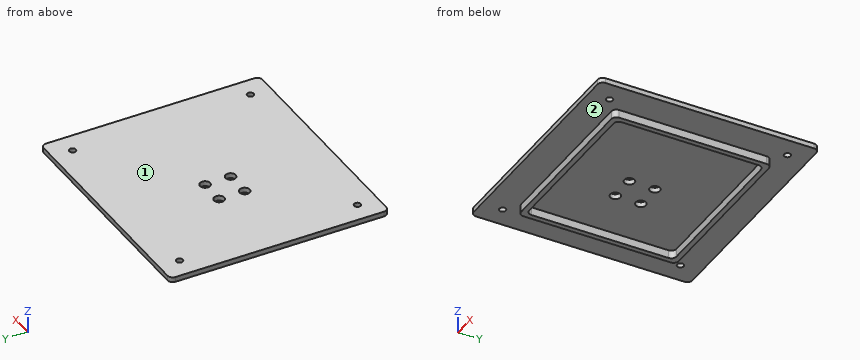
```python
from build123d import *

# Parameters (mm, degrees)
SKETCH_1_W                  = 170
SKETCH_1_H                  = 154.25
SKETCH_1_W_2                = 160
SKETCH_1_H_2                = 144.25
EXTRUDE_1_DEPTH             = 8
FILLET_1_R                  = 5
SKETCH_2_W                  = 230
SKETCH_2_H                  = 214.25
EXTRUDE_2_DEPTH             = 5
FILLET_2_R                  = 5
HOLE_WIZARD_6_4_6_4_1_D     = 6.4
HOLE_WIZARD_6_4_6_4_1_DEPTH = 5
HOLE_WIZARD_10_0_10_1_D     = 10


with BuildPart() as part:
    # 草图1 → 凸台-拉伸1 (new body)
    with BuildSketch(Plane.XY):
        Rectangle(SKETCH_1_W, SKETCH_1_H)
        Rectangle(SKETCH_1_W_2, SKETCH_1_H_2, mode=Mode.SUBTRACT)
    extrude(amount=EXTRUDE_1_DEPTH)

    # 圆角1
    fillet_1_edges = [part.edges().sort_by_distance(p)[0] for p in [
        (-80, 72.125, 4),
        (-80, -72.125, 4),
        (80, -72.125, 4),
        (80, 72.125, 4),
        (-85, 77.125, 4),
        (85, 77.125, 4),
        (85, -77.125, 4),
        (-85, -77.125, 4),
    ]]
    fillet(fillet_1_edges, radius=FILLET_1_R)

    # 草图2 → 凸台-拉伸2 (add)
    with BuildSketch(Plane.XY.offset(8)):
        Rectangle(SKETCH_2_W, SKETCH_2_H)
    extrude(amount=EXTRUDE_2_DEPTH)

    # 圆角2
    fillet_2_edges = [part.edges().sort_by_distance(p)[0] for p in [
        (-115, 107.125, 10.5),
        (-115, -107.125, 10.5),
        (115, -107.125, 10.5),
        (115, 107.125, 10.5),
    ]]
    fillet(fillet_2_edges, radius=FILLET_2_R)

    # Ø6.4 (6.4) 直径孔1
    with Locations(Plane.XY.offset(13)):
        with Locations((-95, 87.125), (95, 87.125), (95, -87.125), (-95, -87.125)):
            Hole(HOLE_WIZARD_6_4_6_4_1_D / 2, depth=HOLE_WIZARD_6_4_6_4_1_DEPTH)

    # Ø10.0 (10) 直径孔1 (through all)
    with Locations(Plane.XY.offset(13)):
        with Locations((-30, 12.5), (-5, 12.5), (-5, -12.5), (-30, -12.5)):
            Hole(HOLE_WIZARD_10_0_10_1_D / 2)


solid = part.part
```
Source: CAD feature listing. Evaluate the final solid. Frame: model axes, mm. Face numbers are marked on the shaded views. A direction names the side the tool comes from. Coordinates: 2 decimals unless noted, no trailing zeros. Write each loop counter-clockwise with the first axis right and the second up, starting at its lowest first coordinate (ties: lowest second). Pieces come first, ordered by that corner, then holes. Notation, with made-up numbers: M -34,3 L 7,3 A22 cw 7,39 Z; hole C 25.25,67.25 d3. An arc over 180 degrees is marked long. Answer as a JSON object with one key per item and string values.
1. Contact query for flat-ended pins moving along their axis: P1, Ø2.5, axis at x = -25.5, z = 3.5, coming from the -Y side (3 decimals); P2, Ø7.5, axis at x = -95, y = 87.125, coming from the -Z side; P3, Ø4, axis at x = -22.5, z = 3.5, coming from the +Y side (3 decimals); P4, Ø4, axis at x = 95, y = 87.125, coming from the +Z side. Output: stop coordinate, or through.
Evaluation:
{"P1": "y = -77.125", "P2": "z = 8", "P3": "y = 77.125", "P4": "through"}
2. Cut plane B-B on y = -12.5. Output: boundary loops of the cut face in (x, z), plus the area to 3 significant figures.
Evaluation:
{"outline": "M -115,8 L -85,8 L -85,0 L -80,0 L -80,8 L -35,8 L -35,13 L -115,13 Z; M -25,8 L -10,8 L -10,13 L -25,13 Z; M 0,8 L 80,8 L 80,0 L 85,0 L 85,8 L 115,8 L 115,13 L 0,13 Z", "area": "1,130 mm^2"}
3. Cut plane A-A on x = -95. Output: boundary loops of the cut face in (y, z) (3 decimals), plus the area to 3 significant figures.
Evaluation:
{"outline": "M -107.125,8 L -90.325,8 L -90.325,13 L -107.125,13 Z; M -83.925,8 L 83.925,8 L 83.925,13 L -83.925,13 Z; M 90.325,8 L 107.125,8 L 107.125,13 L 90.325,13 Z", "area": "1,010 mm^2"}
4. Ray query, L1, parallel to Y at x = -5, z = 11.7 (3 decimals); L2, parallel to Y at x = 95, z = 9.05 (3 decimals); L3, parallel to Y at x = 41, z = 6.5 (3 decimals). Return the intervals inside material, ascending.
Evaluation:
{"L1": "-107.125 to -17.5, -7.5 to 7.5, 17.5 to 107.125", "L2": "-107.125 to -90.325, -83.925 to 83.925, 90.325 to 107.125", "L3": "-77.125 to -72.125, 72.125 to 77.125"}
5. Access query for the marked faces 1 and 2. Directions: +Z, -Z, +X, -X, +Y, -Y. A direction counts if a zero-diameter tool reaches every point of the face in a straight line with its end or side. Return the directions, or none.
Evaluation:
{"face 1": "+Z, +X, -X, +Y, -Y", "face 2": "-Z"}
6. Cut plane C-C on z = 5. Output: boundary loops of the cut face in (x, y) (3 decimals).
Evaluation:
{"outline": "M -85,-72.125 A5 ccw -80,-77.125 L 80,-77.125 A5 ccw 85,-72.125 L 85,72.125 A5 ccw 80,77.125 L -80,77.125 A5 ccw -85,72.125 Z; hole M -80,-67.125 A5 ccw -75,-72.125 L 75,-72.125 A5 ccw 80,-67.125 L 80,67.125 A5 ccw 75,72.125 L -75,72.125 A5 ccw -80,67.125 Z"}
7. Cut plane D-D on y = 43. Output: boundary loops of the cut face in (x, z).
Evaluation:
{"outline": "M -115,8 L -85,8 L -85,0 L -80,0 L -80,8 L 80,8 L 80,0 L 85,0 L 85,8 L 115,8 L 115,13 L -115,13 Z"}
